Model file for the job. Use its own axes, mm. Face numbers are marked on the shaded views. Round coordinates to 2 decimals unless told otherwise and drop trailing zeros. Write each loop counter-clockwise with the first axis right and the second up, starting at its lowest first coordinate (ties: lowest second). Pieces come first, ordered by that corner, then holes. Notation, with made-up numbers: (-6, -8) - (31, -8) arc R12 ccw to (31, 8) - close; hole circle Ø3 at (24.25, 9.25). An arc over 180 degrees is marked (long way). One line per item, written item: value.
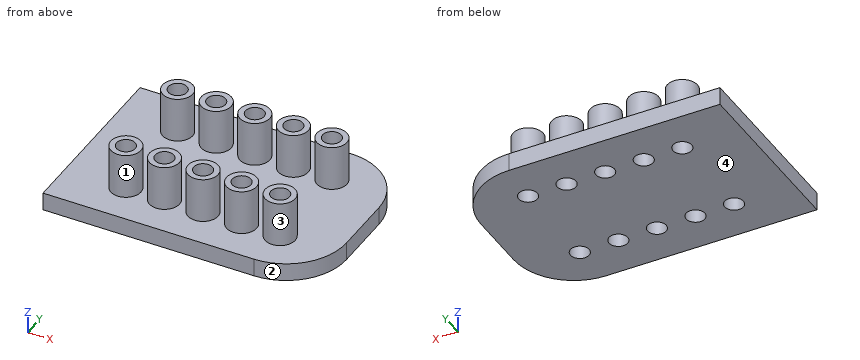
from build123d import *

# Parameters (mm, degrees)
F0_W     = 45
F0_H     = 30
F0_R     = 2.5
F0_R_2   = 1.55
F1_DEPTH = 3
F2_DEPTH = 7.5
F3_R     = 10
F4_ANGLE = 180


with BuildPart() as f1:
    # F0 (on Top) → F1 (new body)
    with BuildSketch(Plane.XY):
        with Locations((22.5, 15)):
            Rectangle(F0_W, F0_H)
        with Locations((10, 7)):
            Circle(F0_R, mode=Mode.SUBTRACT)
        with Locations((16.4, 7)):
            Circle(F0_R, mode=Mode.SUBTRACT)
        with Locations((22.8, 7)):
            Circle(F0_R, mode=Mode.SUBTRACT)
        with Locations((29.2, 7)):
            Circle(F0_R, mode=Mode.SUBTRACT)
        with Locations((35.6, 7)):
            Circle(F0_R, mode=Mode.SUBTRACT)
        with Locations((10, 23)):
            Circle(F0_R, mode=Mode.SUBTRACT)
        with Locations((16.4, 23)):
            Circle(F0_R, mode=Mode.SUBTRACT)
        with Locations((22.8, 23)):
            Circle(F0_R, mode=Mode.SUBTRACT)
        with Locations((29.2, 23)):
            Circle(F0_R, mode=Mode.SUBTRACT)
        with Locations((35.6, 23)):
            Circle(F0_R, mode=Mode.SUBTRACT)
        with Locations((35.6, 23)):
            Circle(F0_R)
        with Locations((35.6, 23)):
            Circle(F0_R_2, mode=Mode.SUBTRACT)
        with Locations((29.2, 23)):
            Circle(F0_R)
        with Locations((29.2, 23)):
            Circle(F0_R_2, mode=Mode.SUBTRACT)
        with Locations((22.8, 23)):
            Circle(F0_R)
        with Locations((22.8, 23)):
            Circle(F0_R_2, mode=Mode.SUBTRACT)
        with Locations((16.4, 23)):
            Circle(F0_R)
        with Locations((16.4, 23)):
            Circle(F0_R_2, mode=Mode.SUBTRACT)
        with Locations((10, 23)):
            Circle(F0_R)
        with Locations((10, 23)):
            Circle(F0_R_2, mode=Mode.SUBTRACT)
        with Locations((10, 7)):
            Circle(F0_R)
        with Locations((10, 7)):
            Circle(F0_R_2, mode=Mode.SUBTRACT)
        with Locations((16.4, 7)):
            Circle(F0_R)
        with Locations((16.4, 7)):
            Circle(F0_R_2, mode=Mode.SUBTRACT)
        with Locations((22.8, 7)):
            Circle(F0_R)
        with Locations((22.8, 7)):
            Circle(F0_R_2, mode=Mode.SUBTRACT)
        with Locations((29.2, 7)):
            Circle(F0_R)
        with Locations((29.2, 7)):
            Circle(F0_R_2, mode=Mode.SUBTRACT)
        with Locations((35.6, 7)):
            Circle(F0_R)
        with Locations((35.6, 7)):
            Circle(F0_R_2, mode=Mode.SUBTRACT)
    extrude(amount=F1_DEPTH)

    # F0 (on Top) → F2 (join)
    with BuildSketch(Plane.XY):
        with Locations((35.6, 23)):
            Circle(F0_R)
        with Locations((35.6, 23)):
            Circle(F0_R_2, mode=Mode.SUBTRACT)
        with Locations((29.2, 23)):
            Circle(F0_R)
        with Locations((29.2, 23)):
            Circle(F0_R_2, mode=Mode.SUBTRACT)
        with Locations((22.8, 23)):
            Circle(F0_R)
        with Locations((22.8, 23)):
            Circle(F0_R_2, mode=Mode.SUBTRACT)
        with Locations((16.4, 23)):
            Circle(F0_R)
        with Locations((16.4, 23)):
            Circle(F0_R_2, mode=Mode.SUBTRACT)
        with Locations((10, 23)):
            Circle(F0_R)
        with Locations((10, 23)):
            Circle(F0_R_2, mode=Mode.SUBTRACT)
        with Locations((10, 7)):
            Circle(F0_R)
        with Locations((10, 7)):
            Circle(F0_R_2, mode=Mode.SUBTRACT)
        with Locations((16.4, 7)):
            Circle(F0_R)
        with Locations((16.4, 7)):
            Circle(F0_R_2, mode=Mode.SUBTRACT)
        with Locations((22.8, 7)):
            Circle(F0_R)
        with Locations((22.8, 7)):
            Circle(F0_R_2, mode=Mode.SUBTRACT)
        with Locations((29.2, 7)):
            Circle(F0_R)
        with Locations((29.2, 7)):
            Circle(F0_R_2, mode=Mode.SUBTRACT)
        with Locations((35.6, 7)):
            Circle(F0_R)
        with Locations((35.6, 7)):
            Circle(F0_R_2, mode=Mode.SUBTRACT)
    extrude(amount=-F2_DEPTH)

    # F3
    f3_edges = [f1.edges().sort_by_distance(p)[0] for p in [
        (45, 30, 1.5),
        (45, 0, 1.5),
    ]]
    fillet(f3_edges, radius=F3_R)


with BuildPart() as f1_1:
    # F4: moved
    add(f1.part.rotate(Axis((22.5, 0, 0), (1, 0, 0)), F4_ANGLE))


solid = f1_1.part
1. Band-saw the part on B-B on z = 5.5. State how many separate pieces and enclosed holes the cut face has, plus the area to 3 significant figures.
Report:
separate pieces: 10
enclosed holes: 10
area: 121 mm²
2. Band-saw the part on A-A on x = 22.8. Write the cut outline in (y, z), plus the area to 3 significant figures.
Report:
outline: (-30, -3) - (-24.55, -3) - (-24.55, 7.5) - (-25.5, 7.5) - (-25.5, 0) - (-30, 0) - close; (-21.45, -3) - (-8.55, -3) - (-8.55, 7.5) - (-9.5, 7.5) - (-9.5, 0) - (-20.5, 0) - (-20.5, 7.5) - (-21.45, 7.5) - close; (-5.45, -3) - (0, -3) - (0, 0) - (-4.5, 0) - (-4.5, 7.5) - (-5.45, 7.5) - close
area: 99.9 mm²
3. Wall check: probe 1 along Y at (x, z) = (22.8, 3.5); probe 2 along Z at (x, y) = (33, -4); probe 3 along Y at (x, z) = (27, 6.5). Give the ranges that are in metal, low to high. Write a range as [from, to].
Report:
probe 1: [-25.5, -24.55], [-21.45, -20.5], [-9.5, -8.55], [-5.45, -4.5]
probe 2: [-3, 0]
probe 3: [-24.19, -21.81], [-8.19, -5.81]
4. Band-saw the part on C-C on x = 35.6. Write the cut outline in (y, z), plus the area to 3 significant figures.
Report:
outline: (-29.98, -3) - (-24.55, -3) - (-24.55, 7.5) - (-25.5, 7.5) - (-25.5, 0) - (-29.98, 0) - close; (-21.45, -3) - (-8.55, -3) - (-8.55, 7.5) - (-9.5, 7.5) - (-9.5, 0) - (-20.5, 0) - (-20.5, 7.5) - (-21.45, 7.5) - close; (-5.45, -3) - (-0.02, -3) - (-0.02, 0) - (-4.5, 0) - (-4.5, 7.5) - (-5.45, 7.5) - close
area: 99.8 mm²
5. Mould opens along Y. For the marked faces 1, 2, 3 and 4 say: released by +Y, released by -Y, zero draft, split by the parting line, or undercut.
Report:
face 1: undercut
face 2: released by -Y
face 3: undercut
face 4: zero draft
